```python
from build123d import *

# Parameters (mm, degrees)
F0_R     = 35
F1_DEPTH = 25
F2_R     = 8.0361334601
F3_DEPTH = 20
F4_R     = 2
F5_R     = 10.3094421679
F6_DEPTH = 25.001
F7_T     = 1.5


with BuildPart() as f1:
    # F0 (on Front) → F1 (new body)
    with BuildSketch(Plane.XZ):
        with BuildLine():
            ThreePointArc((-58.6601695194, -53.7224063011), (-27.590229069, -34.473074379), (-15.4458838051, 0))
            ThreePointArc((-15.4458838051, 0), (-27.590229069, 34.473074379), (-58.6601695194, 53.7224063011))
            ThreePointArc((-58.6601695194, 53.7224063011), (-125.4458838051, 0), (-58.6601695194, -53.7224063011))
        make_face()
        with Locations((-70.4458838051, 0)):
            Circle(F0_R, mode=Mode.SUBTRACT)
        with BuildLine():
            ThreePointArc((-58.6601695194, 53.7224063011), (-27.590229069, 34.473074379), (-15.4458838051, 0))
            ThreePointArc((-15.4458838051, 0), (-27.590229069, -34.473074379), (-58.6601695194, -53.7224063011))
            Line((-58.6601695194, -53.7224063011), (74.9112590521, -24.4192755914))
            ThreePointArc((74.9112590521, -24.4192755914), (44.5541161949, 0), (74.9112590521, 24.4192755914))
            Line((74.9112590521, 24.4192755914), (-58.6601695194, 53.7224063011))
        make_face()
        with BuildLine():
            ThreePointArc((94.5541161949, 0), (89.0339592568, 15.6695792632), (74.9112590521, 24.4192755914))
            ThreePointArc((74.9112590521, 24.4192755914), (44.5541161949, 0), (74.9112590521, -24.4192755914))
            ThreePointArc((74.9112590521, -24.4192755914), (89.0339592568, -15.6695792632), (94.5541161949, 0))
        make_face()
    extrude(amount=F1_DEPTH)

    # F2 (on face) → F3 (join)
    with BuildSketch(Plane(origin=(8.5509543151, 0, 38.9775138646), x_dir=(0.9767710237, 0, -0.2142857143), z_dir=(0.2142857143, 0, 0.9767710237))):
        with Locations((35.0721742403, -12.5)):
            Circle(F2_R)
    extrude(amount=F3_DEPTH)

    # F4
    f4_edges = [f1.edges().sort_by_distance(p)[0] for p in [
        (39.24469, -12.5, 52.719497),
        (34.958976, -12.5, 33.184077),
    ]]
    fillet(f4_edges, radius=F4_R)

    # F5 (on face) → F6 (cut, through all)
    with BuildSketch(Plane.XZ.offset(25)):
        with Locations((69.5541161949, 0)):
            Circle(F5_R)
    extrude(amount=-F6_DEPTH, mode=Mode.SUBTRACT)

    # F7
    f7_openings = [f1.faces().sort_by_distance(p)[0] for p in [
        (-17.192474, -25, 0),
    ]]
    offset(amount=F7_T, openings=f7_openings, kind=Kind.INTERSECTION)


solid = f1.part
```
Geometry check sheet. Reference: the model listing, model coordinates, mm. A direction names the side the tool comes from. Round coordinates to 2 decimals unless told otherwise and drop trailing zeros. Order: outer loops, then holes, each group sorted by start corner. A loop starts at its lowest first (then second) coordinate and runs counter-clockwise, first axis right, second up. Notation, with made-up numbers: (35.25, 17) - (85.25, 17) arc R36 ccw to (85.25, 54) - close; hole circle Ø9 at (1, 43.25). An arc over 180 degrees is marked (long way). Use a Markdown table: item, result. Add a question column.
(1) Material ranges on line 1 along Z through (x, y) = (-40.5, -21); line 2 along Y through (x, z) = (42, 51); line 3 along X through (y, z) = (-21, 22), recorded low to high. Write a range as [from, to].
(2) Sectioned sample at B-B, the plane y = -15. Count the separate pieces of the cut face and the enclosed holes in it, and give its area (3 significant figures).
(3) Sectioned sample at A-A, the plane z = -13. Enter the section's corners in (x, y).
(4) Release check for a two-part mould opening along X. For faces 1 (the flat face through (7.51, -11.56, -40.74)), 2 (the cylindrical face through (77.957, -11.936, 2.646)), 3 (the flat face through (-42, -25, -18)), 4 (the flat face through (7.191, -12.325, -39.276)) record: pulls with the +X half, pulls with the -X half, needs draft (parallel to the pull), parting line crosses it, or undercut.
(5) Tool access check on faces 5 (the flat face through (47.012, -12.415, 51.016)), 6 (the flat face through (1, -25, 42)), 7 (the cylindrical face through (-125.43, -12.32, 1.38)). Record the directions out of +Z, -Z, +X, -X, +Y, -Y that give a thin tool (end or side, any length) a straight path to the whole face; none if there is none.
(6) Depth check by flat-ended pin: pin 1 (1.5 mm diameter, centred on x = -27.5, y = -11, fed in from -Z); pin 2 (8 mm diameter, centred on x = 3.5, y = -15, fed in from -Z); pin 3 (3 mm diameter, centred on y = -14.5, z = 10.5, fed in from -X). Enter the tip coordinate at first touch or a pass-through.
Answers below:
| question | item | result |
|---|---|---|
| 1 | line 1 | [-51.27, -49.74], [-18.12, -15.02], [15.02, 18.12], [49.74, 51.27] |
| 1 | line 2 | [-20.49, -18.53], [-6.47, -4.51] |
| 1 | line 3 | [-122.49, -120.85], [-97.67, -95.71], [-45.18, -43.22], [81.43, 84.33] |
| 2 | separate pieces | 3 |
| 2 | enclosed holes | 3 |
| 2 | area | 1,280 mm² |
| 3 | outline | (-125.43, -25) - (-123.89, -25) - (-123.89, 0) - (-102.94, 0) - (-102.94, -25) - (-101.32, -25) - (-101.32, 1.5) - (-125.43, 1.5) - close; (-39.57, -25) - (-37.95, -25) - (-37.95, 0) - (90.91, 0) - (90.91, -25) - (92.65, -25) - (92.65, 1.5) - (-39.57, 1.5) - close |
| 4 | face 1 | pulls with the +X half |
| 4 | face 2 | undercut |
| 4 | face 3 | needs draft |
| 4 | face 4 | undercut |
| 5 | face 5 | none |
| 5 | face 6 | +Z, -Z, +X, -X, -Y |
| 5 | face 7 | -Y |
| 6 | pin 1 | z = -48.59 |
| 6 | pin 2 | z = -42.5 |
| 6 | pin 3 | x = -126.22 |
